Verification items for this drawing (mm, ordinates from the low corner). Coordinates: 2 decimals unless noted, no trailing zeros. Order: outer loops, then holes, each group sorted by start corner. A loop starts at its lowest first (then second) coordinate and runs counter-clockwise, first axis right, second up.
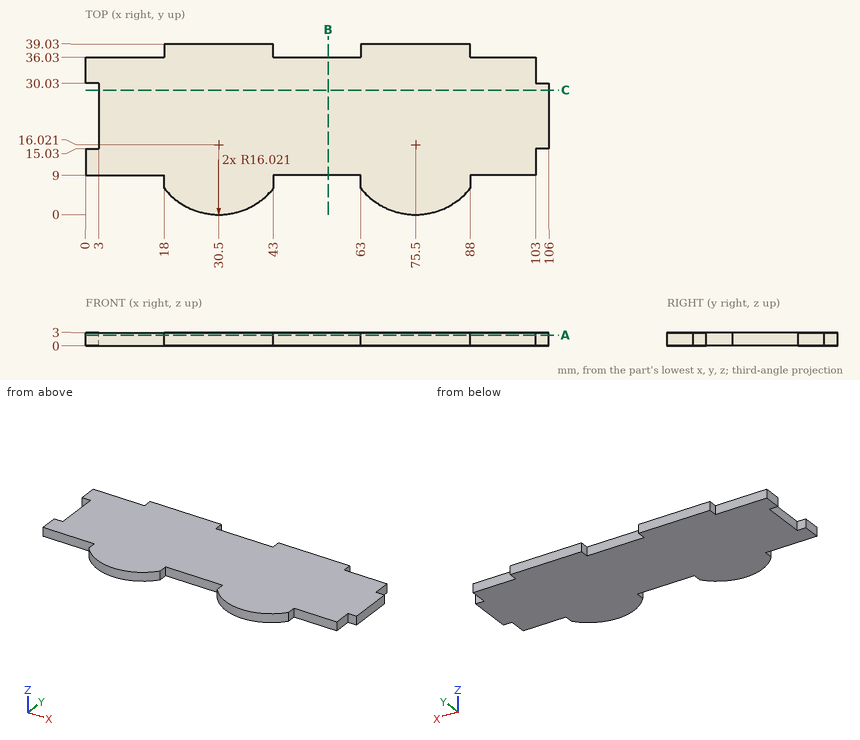
(1) Cross-section at A-A (z = 2.45). Enter the section's corners in (x, y), and give its area (3 significant figures).
Filled in:
outline: (0, 9) - (18, 9) - (18, 6) arc R16.02 ccw to (43, 6) - (43, 9) - (63, 9) - (63, 6) arc R16.02 ccw to (88, 6) - (88, 9) - (103, 9) - (103, 15.03) - (106, 15.03) - (106, 30.03) - (103, 30.03) - (103, 36.03) - (88, 36.03) - (88, 39.03) - (63, 39.03) - (63, 36.03) - (43, 36.03) - (43, 39.03) - (18, 39.03) - (18, 36.03) - (0, 36.03) - (0, 30.03) - (3, 30.03) - (3, 15.03) - (0, 15.03) - close
area: 3,290 mm2
(2) Thickness scan on probe 1 along X at (y, z) = (37, 1.8); probe 2 along X at (y, z) = (32.5, 0.3); probe 3 along Y at (x, z) = (58, 2.65). Record the ranges inside material, lowest first.
Filled in:
probe 1: x = 18 to 43, 63 to 88
probe 2: x = 0 to 103
probe 3: y = 9 to 36.03
(3) Cross-section at C-C (y = 28.5). Enter the section's corners in (x, z), and give its area (3 significant figures).
Filled in:
outline: (3, 0) - (106, 0) - (106, 3) - (3, 3) - close
area: 309 mm2
(4) Cross-section at B-B (x = 55.5). Enter the section's corners in (y, z).
Filled in:
outline: (9, 0) - (36.03, 0) - (36.03, 3) - (9, 3) - close
(5) Go/stop test with flat-tipped pins: P1, Ø1.5, axis at x = 2, z = 2, coming from the -Y side; P2, Ø1.5, axis at y = 38, z = 1, coming from the -X side; P3, Ø0.9, axis at x = 13.5, z = 1, coming from the +Y side. Record where each tip stops, or that it passes through.
Filled in:
P1: stops at y = 9
P2: stops at x = 18
P3: stops at y = 36.03
